CAD build for the part. Positions are in the model's coordinates, mm. A direction names the side the tool comes from. Coordinates: 2 decimals unless noted, no trailing zeros. Write each loop counter-clockwise with the first axis right and the second up, starting at its lowest first coordinate (ties: lowest second). Pieces come first, ordered by that corner, then holes. Notation, with made-up numbers: M 4.5,2.5 L 28.5,2.5 A19 ccw 28.5,22.5 Z; hole C 70,-19 d4. An arc over 180 degrees is marked long. Put each result on its own line as item: value. Start each with the question number.
```python
from build123d import *

# Parameters (mm, degrees)
BOSS_EXTRU_1_DEPTH      = 2
BOSS_EXTRU_3_START      = 25
BOSS_EXTRU_3_DEPTH      = 25
ENL_V_MAT_EXTRU_1_DEPTH = 50


with BuildPart() as part:
    # Esquisse1 → Boss.-Extru.1 (new body)
    with BuildSketch(Plane.XY):
        with BuildLine():
            Line((20, 2), (-20, 2))
            ThreePointArc((-20, 2), (-21.590990258, 1.340990258), (-22.25, -0.25))
            Line((-22.25, -0.25), (-22.25, -19.75))
            ThreePointArc((-22.25, -19.75), (-21.590990258, -21.340990258), (-20, -22))
            Line((-20, -22), (20, -22))
            ThreePointArc((20, -22), (21.590990258, -21.340990258), (22.25, -19.75))
            Line((22.25, -19.75), (22.25, -0.25))
            ThreePointArc((22.25, -0.25), (21.590990258, 1.340990258), (20, 2))
        make_face()
    extrude(amount=BOSS_EXTRU_1_DEPTH)

    # Esquisse2 → Boss.-Extru.3 (add)
    # profile 1 of 2: a face of its own
    with BuildSketch(Plane(origin=(0, 0, 0), x_dir=(-1, 0, 0), z_dir=(0, 0, -1)).offset(BOSS_EXTRU_3_START)):
        with BuildLine():
            Line((-22.25, -19.75), (-22.25, -0.25))
            ThreePointArc((-22.25, -0.25), (-21.590990258, 1.340990258), (-20, 2))
            Line((-20, 2), (20, 2))
            Line((20, 2), (-50, 15))
            Line((-50, 15), (-50, 2))
            Line((-50, 2), (-50, -22))
            Line((-50, -22), (-50, -35))
            Line((-50, -35), (20, -22))
            Line((20, -22), (-20, -22))
            ThreePointArc((-20, -22), (-21.590990258, -21.340990258), (-22.25, -19.75))
        make_face()
    # profile 2 of 2: a face of its own
    with BuildSketch(Plane(origin=(0, 0, 0), x_dir=(-1, 0, 0), z_dir=(0, 0, -1)).offset(BOSS_EXTRU_3_START)):
        with BuildLine():
            Line((20, 2), (-20, 2))
            ThreePointArc((-20, 2), (-21.590990258, 1.340990258), (-22.25, -0.25))
            Line((-22.25, -0.25), (-22.25, -19.75))
            ThreePointArc((-22.25, -19.75), (-21.590990258, -21.340990258), (-20, -22))
            Line((-20, -22), (20, -22))
            ThreePointArc((20, -22), (21.590990258, -21.340990258), (22.25, -19.75))
            Line((22.25, -19.75), (22.25, -0.25))
            ThreePointArc((22.25, -0.25), (21.590990258, 1.340990258), (20, 2))
        make_face()
        with BuildLine():
            ThreePointArc((20.35, -0.25), (20.247487373, -0.002512627), (20, 0.1))
            Line((20, 0.1), (-20, 0.1))
            ThreePointArc((-20, 0.1), (-20.247487373, -0.002512627), (-20.35, -0.25))
            Line((-20.35, -0.25), (-20.35, -19.75))
            ThreePointArc((-20.35, -19.75), (-20.247487373, -19.997487373), (-20, -20.1))
            Line((-20, -20.1), (20, -20.1))
            ThreePointArc((20, -20.1), (20.247487373, -19.997487373), (20.35, -19.75))
            Line((20.35, -19.75), (20.35, -0.25))
        make_face(mode=Mode.SUBTRACT)
    extrude(amount=-BOSS_EXTRU_3_DEPTH)

    # Esquisse5 → Enlèv. mat.-Extru.1 (cut)
    with BuildSketch(Plane(origin=(0, 0, -25), x_dir=(-1, 0, 0), z_dir=(0, 0, -1))):
        Polygon((-22.26420213, 7.916578551), (-48.1, 12.714655299), (-48.1, -32.714655299), (-22.26420213, -27.916578551), align=None)
    extrude(amount=-ENL_V_MAT_EXTRU_1_DEPTH, mode=Mode.SUBTRACT)


solid = part.part
```
(1) Drill centre lines: line 1 (X direction, y = -16, z = -15); line 2 (X direction, y = 0, z = -20.25); line 3 (X direction, y = -7.5, z = 0.25). Where is each one in solid material? Low to high. Write a range as [from, to].
(2) Which spindle directions (+Z, -Z, +X, -X, +Y, -Y) get a long thin tool onto all of the face, cutting with end or side? Do faces 4 (the face through (21.57, -21.36, 0.99)), 5 (the face through (0, 0.1, -13)), 6 (the face through (35.36, -30.35, -12.68)), 7 (the face through (0, -22, 1)). Say none if no direction does.
(3) Slice it at D-D, the plane y = 4. Write the cut outline in (x, z).
(4) Two-plate mould, pull along X, no slides. Class faces 1 (the face through (-21.61, 1.32, -11.69)), 2 (the face through (22.25, -10, 1)), 3 (the face through (-20.35, -10, -13)): +X half, -X half, draft (parallel to the pull), parting line (faces both ways), or undercut.
(5) Slice it at C-C, the plane x = -14. Write the cut outline in (y, z).
(6) Drop flat-ended pins along their axis: pin 1 (6 mm diameter, centred on x = -2.5, y = -5.5, fed in from -Z); pin 2 (1.5 mm diameter, centred on x = 31, y = -29, fed in from +Z); pin 3 (5 mm diameter, centred on x = 0, z = -13.5, fed in from -Y). Give the stop position or say it passes through.
(7) Slice it at A-A, the plane z = -1.5. Write the cut outline in (x, y), then the cut area to 3 significant figures.
Result set:
1. line 1: x = [-22.25, -20.35], [20.35, 22.26], [48.1, 50]
1. line 2: x = [-22.24, -20.24], [20.24, 22.26], [48.1, 50]
1. line 3: x = [-22.25, 22.25]
2. face 4: +Z, +X, -Y
2. face 5: -Z
2. face 6: +Z, -Z
2. face 7: +Z, +X, -X, -Y
3. outline: M -9.23,-25 L 22.26,-25 L 22.26,0 L -9.23,0 Z; M 48.1,-25 L 50,-25 L 50,0 L 48.1,0 Z
4. face 1: -X half
4. face 2: +X half
4. face 3: undercut
5. outline: M -23.11,-25 L -20.1,-25 L -20.1,0 L 0.1,0 L 0.1,-25 L 3.11,-25 L 3.11,0 L 2,0 L 2,2 L -22,2 L -22,0 L -23.11,0 Z
6. pin 1: stops at z = 0
6. pin 2: stops at z = 0
6. pin 3: stops at y = -26.18
7. outline: M -22.25,-19.75 A2.25 ccw -20,-22 L 50,-35 L 50,15 L -20,2 A2.25 ccw -22.25,-0.25 Z; hole M -20.35,-19.75 A0.35 ccw -20,-20.1 L 20,-20.1 A0.35 ccw 20.35,-19.75 L 20.35,-0.25 A0.35 ccw 20,0.1 L -20,0.1 A0.35 ccw -20.35,-0.25 Z; hole M 22.26,-27.92 L 48.1,-32.71 L 48.1,12.71 L 22.26,7.92 Z
7. area: 770 mm^2
